```python
from build123d import *

# Parameters (mm, degrees)
CUT_EXTRUDE2_START = -100
CUT_EXTRUDE2_DEPTH = 100


with BuildPart() as part:
    # Sketch1 → Revolve1 (revolve)
    with BuildSketch(Plane.XY, mode=Mode.PRIVATE) as revolve1_sk:
        Polygon((25, 24), (25, 4.595744681), (25, 0), (11, 0), (11, 7), (6, 7), (6, 17), (11, 17), (11, 24), align=None)
    revolve(revolve1_sk.sketch.rotate(Axis((0, 0, 0), (0, 1, 0)), 90), axis=Axis((0, 0, 0), (0, 1, 0)))

    # Sketch2 → Cut-Extrude2 (cut)
    with BuildSketch(Plane(origin=(0, 24, 0), x_dir=(1, 0, 0), z_dir=(0, 1, 0)).offset(CUT_EXTRUDE2_START)):
        with BuildLine():
            Line((4.341204442, 24.620193825), (2.604722665, 14.772116295))
            ThreePointArc((2.604722665, 14.772116295), (10.606601718, 10.606601718), (14.772116295, 2.604722665))
            Line((14.772116295, 2.604722665), (24.620193825, 4.341204442))
            ThreePointArc((24.620193825, 4.341204442), (17.67766953, 17.67766953), (4.341204442, 24.620193825))
        make_face()
        with BuildLine():
            ThreePointArc((15, 0), (14.942920471, -1.307336141), (14.772116295, -2.604722665))
            Line((14.772116295, -2.604722665), (24.620193825, -4.341204442))
            ThreePointArc((24.620193825, -4.341204442), (24.904867452, -2.178893569), (25, 0))
            ThreePointArc((25, 0), (24.904867452, 2.178893569), (24.620193825, 4.341204442))
            Line((24.620193825, 4.341204442), (14.772116295, 2.604722665))
            ThreePointArc((14.772116295, 2.604722665), (14.942920471, 1.307336141), (15, 0))
        make_face()
        with BuildLine():
            Line((24.620193825, -4.341204442), (14.772116295, -2.604722665))
            ThreePointArc((14.772116295, -2.604722665), (10.606601718, -10.606601718), (2.604722665, -14.772116295))
            Line((2.604722665, -14.772116295), (4.341204442, -24.620193825))
            ThreePointArc((4.341204442, -24.620193825), (17.67766953, -17.67766953), (24.620193825, -4.341204442))
        make_face()
        with BuildLine():
            Line((-4.341204442, -24.620193825), (-2.604722665, -14.772116295))
            ThreePointArc((-2.604722665, -14.772116295), (-10.606601718, -10.606601718), (-14.772116295, -2.604722665))
            Line((-14.772116295, -2.604722665), (-24.620193825, -4.341204442))
            ThreePointArc((-24.620193825, -4.341204442), (-17.67766953, -17.67766953), (-4.341204442, -24.620193825))
        make_face()
        with BuildLine():
            ThreePointArc((-14.772116295, -2.604722665), (-15, 0), (-14.772116295, 2.604722665))
            Line((-14.772116295, 2.604722665), (-24.620193825, 4.341204442))
            ThreePointArc((-24.620193825, 4.341204442), (-25, 0), (-24.620193825, -4.341204442))
            Line((-24.620193825, -4.341204442), (-14.772116295, -2.604722665))
        make_face()
        with BuildLine():
            ThreePointArc((-14.772116295, 2.604722665), (-10.606601718, 10.606601718), (-2.604722665, 14.772116295))
            Line((-2.604722665, 14.772116295), (-4.341204442, 24.620193825))
            ThreePointArc((-4.341204442, 24.620193825), (-17.67766953, 17.67766953), (-24.620193825, 4.341204442))
            Line((-24.620193825, 4.341204442), (-14.772116295, 2.604722665))
        make_face()
    extrude(amount=CUT_EXTRUDE2_DEPTH, mode=Mode.SUBTRACT)


solid = part.part
```
Input: part model. Units: mm. Frame: model coordinates. A direction names the side the tool comes from. Coordinates: 2 decimals unless noted, no trailing zeros. Write each loop counter-clockwise with the first axis right and the second up, starting at its lowest first coordinate (ties: lowest second). Pieces come first, ordered by that corner, then holes. Notation, with made-up numbers: (81.5, 88) -> (88.5, 88) arc R26 cw to (88.5, 105) -> close; hole circle Ø2 at (-22, 59). An arc over 180 degrees is marked (long way). Answer as a JSON object with one key per item and string values.
1. Section A-A on x = 0. Return the cut outline in (y, z), then the cut area to 3 significant figures.
Result set:
{"outline": "(0, -25) -> (24, -25) -> (24, -11) -> (17, -11) -> (17, -6) -> (7, -6) -> (7, -11) -> (0, -11) -> close; (0, 11) -> (7, 11) -> (7, 6) -> (17, 6) -> (17, 11) -> (24, 11) -> (24, 25) -> (0, 25) -> close", "area": "772 mm2"}
2. Section D-D on x = 7. Return the cut outline in (y, z), then the cut area to 3 significant figures.
Result set:
{"outline": "(0, -13.27) -> (24, -13.27) -> (24, -8.49) -> (17, -8.49) -> (17, 8.49) -> (24, 8.49) -> (24, 13.27) -> (0, 13.27) -> (0, 8.49) -> (7, 8.49) -> (7, -8.49) -> (0, -8.49) -> close", "area": "399 mm2"}
3. Mould query, pull axis X, two halves, no side actions, for faces 4 (the face through (10.74, 20.55, 2.38)), 5 (the face through (11, 0, 2)), 6 (the face through (10.74, 3.55, 2.38)), 7 (the face through (0, 12, -25)). Classes: released by +X, released by -X, zero draft, split by the parting line, or undercut.
Result set:
{"face 4": "undercut", "face 5": "zero draft", "face 6": "undercut", "face 7": "split by the parting line"}
4. First-contact query: P1, Ø17.5, axis at x = 1, z = 1.5, coming from the -Y side; P2, Ø17.5, axis at x = 0, z = 0, coming from the +Y side; P3, Ø1.5, axis at x = -6, y = 15.5, coming from the +Z side. Flat tips, straight axial feed; report the tip coordinate or a pass-through.
Result set:
{"P1": "stops at y = 7", "P2": "stops at y = 17", "P3": "stops at z = 14.05"}
5. Section B-B on y = 12.5. Return the cut outline in (x, z).
Result set:
{"outline": "(-4.34, -24.62) arc R25 ccw to (4.34, -24.62) -> (2.6, -14.77) arc R15 ccw to (2.6, 14.77) -> (4.34, 24.62) arc R25 ccw to (-4.34, 24.62) -> (-2.6, 14.77) arc R15 ccw to (-2.6, -14.77) -> close; hole circle Ø12 at (0, 0)"}
6. Material intervals for line 1 (Y direction, x = 4.5, z = -9); line 2 (Z direction, x = 8, y = 4.5); line 3 (Z direction, x = 2.5, y = 19), sorted ascending. Write a range as from..to.
Result set:
{"line 1": "y = 7..17", "line 2": "z = -12.69..-7.55, 7.55..12.69", "line 3": "z = -24.87..-10.71, 10.71..24.87"}
7. Access query for faces 1 (the face through (-3.46, 11.83, -19.63)), 2 (the face through (5, 17, 5)), 3 (the face through (3.485, 11.832, -19.765)). Directions: +Z, -Z, +X, -X, +Y, -Y. A direction counts if a zero-diameter tool reaches every point of the face in a straight line with its end or side. Return the directions, or none.
Result set:
{"face 1": "-X, +Y, -Y", "face 2": "+Y", "face 3": "+X, +Y, -Y"}
8. Section C-C on z = 3.5. Return the cut outline in (x, y).
Result set:
{"outline": "(-14.59, 0) -> (-10.43, 0) -> (-10.43, 7) -> (-4.87, 7) -> (-4.87, 17) -> (-10.43, 17) -> (-10.43, 24) -> (-14.59, 24) -> close; (4.87, 7) -> (10.43, 7) -> (10.43, 0) -> (14.59, 0) -> (14.59, 24) -> (10.43, 24) -> (10.43, 17) -> (4.87, 17) -> close"}
